The listing builds one solid part. Answer for the finished solid, in the listing's coordinates (mm). A direction names the side the tool comes from. Round coordinates to 2 decimals unless told otherwise and drop trailing zeros. Loops run counter-clockwise (first coordinate to the right, second up) from the corner with the lowest first, then second, coordinate; pieces in that order, holes last. Notation, with made-up numbers: (70, 31) -> (118, 31) arc R23 cw to (118, 68) -> close; hole circle Ø9 at (8.25, 26.5). An arc over 180 degrees is marked (long way). Answer in a Markdown table with one row per item. Add a question column.
```python
from build123d import *

# Parameters (mm, degrees)
EXTRUDE_1_DEPTH     = 3
SKETCH_4_W          = 3
SKETCH_4_H          = 3
EXTRUDE_2_DEPTH     = 8
SKETCH_5_W          = 3
SKETCH_5_H          = 3
EXTRUDE_3_DEPTH     = 17
SKETCH_6_R          = 5
CUT_EXTRUDE_1_DEPTH = 2


with BuildPart() as part:
    # 草图1 → 凸台-拉伸1 (new body)
    with BuildSketch(Plane.XY):
        Polygon((2.5, 0), (0, -10), (-3, -10), (-3, -30), (0, -30), (20, -30), (23, -30), (23, -10), (20, -10), (17.5, 0), align=None)
    extrude(amount=EXTRUDE_1_DEPTH)

    # 草图4 → 凸台-拉伸2 (add)
    with BuildSketch(Plane(origin=(0, 0, 0), x_dir=(-1, 0, 0), z_dir=(0, 0, -1))):
        with Locations((-21.5, -11.5)):
            Rectangle(SKETCH_4_W, SKETCH_4_H)
        with Locations((1.5, -11.5)):
            Rectangle(SKETCH_4_W, SKETCH_4_H)
    extrude(amount=EXTRUDE_2_DEPTH)

    # 草图5 → 凸台-拉伸3 (add)
    with BuildSketch(Plane.XZ.offset(13)):
        with Locations((-1.5, -6.5)):
            Rectangle(SKETCH_5_W, SKETCH_5_H)
        with Locations((21.5, -6.5)):
            Rectangle(SKETCH_5_W, SKETCH_5_H)
    extrude(amount=EXTRUDE_3_DEPTH)

    # 草图6 → 切除-拉伸1 (cut)
    with BuildSketch(Plane(origin=(0, 0, 0), x_dir=(-1, 0, 0), z_dir=(0, 0, -1))):
        with Locations((-10, -20)):
            Circle(SKETCH_6_R)
    extrude(amount=-CUT_EXTRUDE_1_DEPTH, mode=Mode.SUBTRACT)


solid = part.part
```
Item 1: Section B-B, the plane y = -20 is taken. Write down the section's boundary in (x, z), and give its area (3 significant figures).
Item 2: The mould has two halves that part along X. Classify faces 4 (the flat face through (10, -20, 2)), 5 (the flat face through (10, 0, 1)), 6 (the flat face through (1.267, -4.93, 1.479)): +X half, -X half, draft (parallel to the pull), parting line (faces both ways), or undercut.
Item 3: Flat-ended cylindrical pins translate along their axes: P1, Ø0.9, axis at x = 21.5, z = -1.5, coming from the -Y side; P2, Ø11, axis at x = 11, y = -21.5, coming from the -Z side; P3, Ø1.5, axis at x = -1, z = -4.5, coming from the +Y side. Find the tip coordinate at first contact, or state that the pin passes through.
Item 4: Section A-A, the plane z = -1 is taken. Write down the section's boundary in (x, y), and give its area (3 significant figures).
Item 5: Section C-C, the plane z = 1 is taken. Write down the section's boundary in (x, y), and give its area (3 significant figures).
Item 6: Section D-D, the plane x = 10 is taken. Write down the section's boundary in (y, z).
Item 7: Consider L1, parallel to Y at x = 10, z = 1; L2, parallel to X at y = -12.5, z = -0.25; L3, parallel to Z at x = 15.25, y = -8. Determine where each line is inside the solid, lowest interval first. Write a range as from..to.
Item 8: For faces 1 (the flat face through (-1, -13, -2)), 2 (the flat face through (22, -10, -2)), 3 (the cylindrical face through (7.693, -24.436, 0.986)), determine the directions among +Z, -Z, +X, -X, +Y, -Y from which every point of the face is accessible in a straight line to the end or side of a thin tool.
Here are the results:
| question | item | result |
|---|---|---|
| 1 | outline | (-3, -8) -> (0, -8) -> (0, -5) -> (-3, -5) -> close; (-3, 0) -> (5, 0) -> (5, 2) -> (15, 2) -> (15, 0) -> (23, 0) -> (23, 3) -> (-3, 3) -> close; (20, -8) -> (23, -8) -> (23, -5) -> (20, -5) -> close |
| 1 | area | 76.0 mm² |
| 2 | face 4 | undercut |
| 2 | face 5 | draft |
| 2 | face 6 | -X half |
| 3 | P1 | stops at y = -13 |
| 3 | P2 | stops at z = 0 |
| 3 | P3 | stops at y = -10 |
| 4 | outline | (-3, -13) -> (0, -13) -> (0, -10) -> (-3, -10) -> close; (20, -13) -> (23, -13) -> (23, -10) -> (20, -10) -> close |
| 4 | area | 18.0 mm² |
| 5 | outline | (-3, -30) -> (23, -30) -> (23, -10) -> (20, -10) -> (17.5, 0) -> (2.5, 0) -> (0, -10) -> (-3, -10) -> close; hole circle Ø10 at (10, -20) |
| 5 | area | 616 mm² |
| 6 | outline | (-30, 0) -> (-25, 0) -> (-25, 2) -> (-15, 2) -> (-15, 0) -> (0, 0) -> (0, 3) -> (-30, 3) -> close |
| 7 | L1 | y = -30..-25, -15..0 |
| 7 | L2 | x = -3..0, 20..23 |
| 7 | L3 | z = 0..3 |
| 8 | face 1 | +X, -X, -Y |
| 8 | face 2 | +Z, -Z, +X, +Y |
| 8 | face 3 | -Z |
